from build123d import *

# Parameters (mm, degrees)
SKETCH1_R           = 35.1
SKETCH1_R_2         = 2.1
SKETCH1_R_3         = 15
MAIN_BODY_DEPTH     = 10
CHAMFER3_SIZE       = 0.5
CHAMFER4_SIZE       = 1
BOSS_EXTRUDE4_START = -6
SKETCH2_R           = 15
SKETCH2_R_2         = 12.5
BOSS_EXTRUDE4_DEPTH = 6
CUT_EXTRUDE1_DEPTH  = 2.5


with BuildPart() as part:
    # Sketch1 → Main Body (new body)
    with BuildSketch(Plane(origin=(0, 0, 0), x_dir=(1, 0, 0), z_dir=(0, 1, 0))):
        with Locations(Location((0, 0, 0), (0, 0, 270))):
            Circle(SKETCH1_R)
        with Locations(Location((0, 30, 0), (0, 0, 270))):
            Circle(SKETCH1_R_2, mode=Mode.SUBTRACT)
        with Locations(Location((25.980762114, 15, 0), (0, 0, 270))):
            Circle(SKETCH1_R_2, mode=Mode.SUBTRACT)
        with Locations(Location((25.980762114, -15, 0), (0, 0, 270))):
            Circle(SKETCH1_R_2, mode=Mode.SUBTRACT)
        with Locations(Location((0, -30, 0), (0, 0, 270))):
            Circle(SKETCH1_R_2, mode=Mode.SUBTRACT)
        with Locations(Location((-25.980762114, -15, 0), (0, 0, 270))):
            Circle(SKETCH1_R_2, mode=Mode.SUBTRACT)
        with Locations(Location((-25.980762114, 15, 0), (0, 0, 270))):
            Circle(SKETCH1_R_2, mode=Mode.SUBTRACT)
        with Locations(Location((0, 0, 0), (0, 0, 270))):
            Circle(SKETCH1_R_3, mode=Mode.SUBTRACT)
    extrude(amount=MAIN_BODY_DEPTH)

    # Chamfer3
    chamfer3_edges = [part.edges().sort_by_distance(p)[0] for p in [
        (25.980762114, 10, -17.1),
        (25.980762114, 10, 12.9),
        (0, 10, 27.9),
        (-25.980762114, 10, 12.9),
        (-25.980762114, 10, -17.1),
        (0, 10, -32.1),
    ]]
    chamfer(chamfer3_edges, length=CHAMFER3_SIZE)

    # Chamfer4
    chamfer4_edges = [part.edges().sort_by_distance(p)[0] for p in [
        (0, 0, -15),
    ]]
    chamfer(chamfer4_edges, length=CHAMFER4_SIZE)

    # Sketch2 → Boss-Extrude4 (add)
    with BuildSketch(Plane(origin=(0, 10, 0), x_dir=(1, 0, 0), z_dir=(0, 1, 0)).offset(BOSS_EXTRUDE4_START)):
        with Locations(Location((0, 0, 0), (0, 0, 270))):
            Circle(SKETCH2_R)
        with Locations(Location((0, 0, 0), (0, 0, 270))):
            Circle(SKETCH2_R_2, mode=Mode.SUBTRACT)
    extrude(amount=BOSS_EXTRUDE4_DEPTH)

    # Sketch3 → Cut-Extrude1 (cut)
    with BuildSketch(Plane.XZ):
        Polygon((25.980762114, 10.958548116), (29.480762114, 12.979274058), (29.480762114, 17.020725942), (25.980762114, 19.041451884), (22.480762114, 17.020725942), (22.480762114, 12.979274058), align=None)
        Polygon((0, 25.958548116), (3.5, 27.979274058), (3.5, 32.020725942), (0, 34.041451884), (-3.5, 32.020725942), (-3.5, 27.979274058), align=None)
        Polygon((22.480762114, -17.020725942), (25.980762114, -19.041451884), (29.480762114, -17.020725942), (29.480762114, -12.979274058), (25.980762114, -10.958548116), (22.480762114, -12.979274058), align=None)
        Polygon((-3.5, -27.979274058), (-3.5, -32.020725942), (0, -34.041451884), (3.5, -32.020725942), (3.5, -27.979274058), (0, -25.958548116), align=None)
        Polygon((-25.980762114, -10.958548116), (-29.480762114, -12.979274058), (-29.480762114, -17.020725942), (-25.980762114, -19.041451884), (-22.480762114, -17.020725942), (-22.480762114, -12.979274058), align=None)
        Polygon((-22.480762114, 17.020725942), (-25.980762114, 19.041451884), (-29.480762114, 17.020725942), (-29.480762114, 12.979274058), (-25.980762114, 10.958548116), (-22.480762114, 12.979274058), align=None)
    extrude(amount=-CUT_EXTRUDE1_DEPTH, mode=Mode.SUBTRACT)


solid = part.part
Design review of the part built by this model. Coordinates are the model's own, in mm. A direction names the side the tool comes from. Coordinates: 2 decimals unless noted, no trailing zeros. Loops run counter-clockwise (first coordinate to the right, second up) from the corner with the lowest first, then second, coordinate; pieces in that order, holes last. Notation, with made-up numbers: M 33.25,-23.5 L 81.25,-23.5 A21 ccw 81.25,-2.5 Z; hole C 64,52.25 d5. An arc over 180 degrees is marked long. Answer as CSV lines item,"result".
Item 1: The part is to be moulded in two halves that separate along X. For faces 3 (the face through (-15, 0, 7)), 4 (the face through (27.755, 1.232, 18.017)), say which applies: pulls with the +X half, pulls with the -X half, needs draft (parallel to the pull), parting line crosses it, or undercut.
Answer list:
face 3,"needs draft"
face 4,"undercut"
Item 2: Add section C-C on z = -30. State the section outline as (x, y) points, plus the area to 3 significant figures.
Answer list:
outline,"M -18.22,0 L -3.5,0 L -3.5,2.5 L -2.1,2.5 L -2.1,9.5 L -2.6,10 L -18.22,10 Z; M 2.1,2.5 L 3.5,2.5 L 3.5,0 L 18.22,0 L 18.22,10 L 2.6,10 L 2.1,9.5 Z"
area,"315 mm²"
Item 3: For P1, Ø4, axis at y = 5.5, z = 18.5, coming from the +X side; P2, Ø0.8, axis at y = 2, z = 15.5, coming from the -X side; P3, Ø0.8, axis at y = 1, z = -15.5, coming from the +X side, all flat-tipped, find the tip position at first contact; note any pin that passes through.
Answer list:
P1,"x = 30.98"
P2,"x = -31.69"
P3,"x = 31.69"
Item 4: Machinability: for faces 1 (the face through (1.726, 1.232, -33.045)), 2 (the face through (-1.278, 5.951, -31.666)), which of the approach directions +Z, -Z, +X, -X, +Y, -Y give a long, thin tool a straight path to every point of the face, cutting with its end or side? Answer none if there is none.
Answer list:
face 1,"-Y"
face 2,"+Y, -Y"
Item 5: Add section A-A on z = 0. State the section outline as (x, y) points.
Answer list:
outline,"M -35.1,0 L -16,0 L -15,1 L -15,4 L -12.5,4 L -12.5,10 L -35.1,10 Z; M 12.5,4 L 15,4 L 15,1 L 16,0 L 35.1,0 L 35.1,10 L 12.5,10 Z"
Item 6: For probe 1 along X at (y, z) = (5, -15); probe 2 along Z at (x, y) = (1.5, 9.25); probe 3 along Z at (x, y) = (11.5, 4.25), list the stretches that pass through material, from the lowest coordinate up.
Answer list:
probe 1,"-31.73 to -28.08, -23.88 to 23.88, 28.08 to 31.73"
probe 2,"-35.07 to -31.47, -28.53 to -12.41, 12.41 to 28.53, 31.47 to 35.07"
probe 3,"-33.16 to -4.9, 4.9 to 33.16"
Item 7: Add section D-D on z = 20. State the section outline as (x, y) points.
Answer list:
outline,"M -28.84,0 L 28.84,0 L 28.84,10 L -28.84,10 Z"
Item 8: Add section B-B on y = 5.75. State the section outline as (x, z) points.
Answer list:
outline,"C 0,0 d70.2; hole C -25.98,-15 d4.2; hole C -25.98,15 d4.2; hole C 0,0 d25; hole C 0,-30 d4.2; hole C 0,30 d4.2; hole C 25.98,-15 d4.2; hole C 25.98,15 d4.2"
